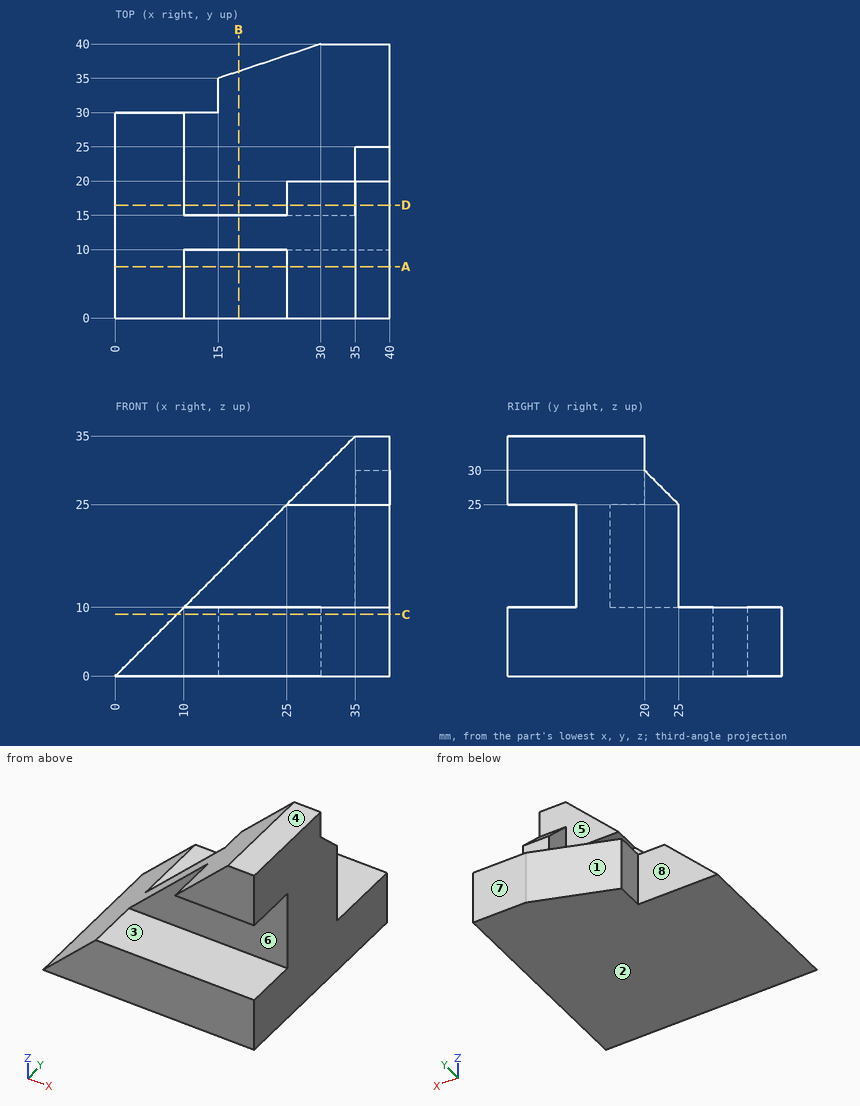
Geometry check sheet. Reference: drawing and pictorial views, mm from the part's lowest x, y, z. A direction names the side the tool comes from. Coordinates: 2 decimals unless noted, no trailing zeros. Order: outer loops, then holes, each group sorted by start corner. A loop starts at its lowest first (then second) coordinate and runs counter-clockwise, first axis right, second up. Notation, with made-up numbers: M 40,-28.75 L 81,-28.75 A26 cw 81,-11.75 Z; hole C -29,66.5 d9. An arc over 180 degrees is marked long. Return JSON: item names as keys, results as strings.
1) Release check for a two-part mould opening along Z. For the marked faces 1, 2, 3 and 4 record: +Z half, -Z half, draft (parallel to the pull), parting line (faces both ways), or undercut.
Answer list:
{"face 1": "draft", "face 2": "-Z half", "face 3": "undercut", "face 4": "+Z half"}
2) Gauge pin test, flat ends, axial feed: pin 1 (1 mm diameter, centred on x = 18, y = 5.5, fed in from +Z); pin 2 (2 mm diameter, centred on y = 21.5, z = 31, fed in from +X); pin 3 (3 mm diameter, centred on x = 17.5, z = 8.5, fed in from +Y); pin 4 (8 mm diameter, centred on y = 20, z = 19, fed in from -X). Record the tip position at first contact, or that the pin passes through.
Answer list:
{"pin 1": "z = 10", "pin 2": "through", "pin 3": "y = 36.33", "pin 4": "x = 35"}
3) Cross-section at A-A, the plane y = 7.5. Record the boundary of the cut face in (x, z).
Answer list:
{"outline": "M 0,0 L 40,0 L 40,10 L 10,10 Z; M 25,25 L 40,25 L 40,35 L 35,35 Z"}
4) Cross-section at D-D, the plane y = 16.5. Record the boundary of the cut face in (x, z).
Answer list:
{"outline": "M 0,0 L 40,0 L 40,35 L 35,35 L 25,25 L 35,25 L 35,10 L 10,10 Z"}
5) Cross-section at C-C, the plane z = 9. Record the boundary of the cut face in (x, y), and give its area (3 significant figures).
Answer list:
{"outline": "M 9,0 L 40,0 L 40,40 L 30,40 L 15,35 L 15,30 L 9,30 Z", "area": "1,140 mm2"}
6) Access from +Z, -Z, +X, -X, +Y, -Y to the whole of each face (thin tool, end or side, straight path). Record for the marked faces 5, 6, 7 and 8.
Answer list:
{"face 5": "+Z, -X, +Y", "face 6": "+X, -X, -Y", "face 7": "+Z, -Z, +X, -X, +Y", "face 8": "+Z, -Z, -X, +Y"}
7) Thickness scan on L1, parallel to Z at x = 18, y = 32.5; L2, parallel to X at y = 19.5, z = 12; L3, parallel to Y at x = 38, z = 22.5. Record the ranges inside material, lowest first. Write a range as [from, to].
Answer list:
{"L1": "[0, 10]", "L2": "[35, 40]", "L3": "[10, 25]"}
8) Cross-section at B-B, the plane x = 18. Record the boundary of the cut face in (y, z), and give its area (3 significant figures).
Answer list:
{"outline": "M 0,0 L 36,0 L 36,10 L 15,10 L 15,18 L 10,18 L 10,10 L 0,10 Z", "area": "400 mm2"}
